from build123d import *

# Parameters (mm, degrees)
BOSS_EXTRUDE1_DEPTH        = 3
F_10_0MM_DOWEL_HOLE1_D     = 10
F_10_0MM_DOWEL_HOLE1_DEPTH = 3
F_3_0MM_DOWEL_HOLE1_D      = 3
F_3_0MM_DOWEL_HOLE1_DEPTH  = 3


with BuildPart() as part:
    # Sketch1 → Boss-Extrude1 (new body)
    with BuildSketch(Plane(origin=(0, 0, 0), x_dir=(1, 0, 0), z_dir=(0, 1, 0))):
        Polygon((-13.2, 0), (180, 0), (150.720058283, 100), (16.079941717, 100), align=None)
    extrude(amount=BOSS_EXTRUDE1_DEPTH)

    # Ø10.0mm Dowel Hole1
    with Locations(Plane(origin=(0, 3, 0), x_dir=(1, 0, 0), z_dir=(0, 1, 0))):
        with Locations((83.4, 50)):
            Hole(F_10_0MM_DOWEL_HOLE1_D / 2, depth=F_10_0MM_DOWEL_HOLE1_DEPTH)

    # Ø3.0mm Dowel Hole1
    with Locations(Plane(origin=(0, 3, 0), x_dir=(1, 0, 0), z_dir=(0, 1, 0))):
        with Locations((73.45, 58.95), (73.45, 41.05), (93.35, 41.05), (93.35, 58.95)):
            Hole(F_3_0MM_DOWEL_HOLE1_D / 2, depth=F_3_0MM_DOWEL_HOLE1_DEPTH)


solid = part.part
Model file for the job. Use its own axes, mm. Give positions to 0.01 mm unless a question says otherwise; leave off trailing zeros. Order: outer loops, then holes, each group sorted by start corner. A loop starts at its lowest first (then second) coordinate and runs counter-clockwise, first axis right, second up. Notation, with made-up numbers: (53.5, -34) - (109.5, -34) arc R21 cw to (109.5, -15) - close; hole circle Ø1 at (-12.75, 76.25). An arc over 180 degrees is marked (long way). Write item = value, one per line. Start each with the question number.
1. Probe line 1 along Z through (x, y) = (73.45, 1.7); line 2 along X through (y, z) = (1.25, -41.05); line 3 along Z through (x, y) = (83.4, 1.15). List the from-to ranges inside material, lowest first.
2. Two-plate mould, pull along Z, no slides. Class faces 1 (the flat face through (1.645, 1.479, -50.7)), 2 (the flat face through (82, 0, -40)), 3 (the cylindrical face through (80.712, 1.479, -54.216)): pulls with the +Z half, pulls with the -Z half, needs draft (parallel to the pull), parting line crosses it, or undercut.
3. Cut at A-A, the plane y = 0.5. List the corners of the cut face in (x, z).
4. Drop a flat-ended pin along its axis: P1, Ø1.8, axis at x = 73.45, z = -58.95, coming from the -Y side. Give the stop position or say it passes through.
5. Cut at C-C, the plane z = -75. List the corners of the cut face in (x, y).
6. Cut at B-B, the plane z = -50. List the corners of the cut face in (x, y).
Taken from the geometry:
q1.line_1 = -100 to -60.45, -57.45 to -42.55, -39.55 to 0
q1.line_2 = -1.18 to 71.95, 74.95 to 91.85, 94.85 to 167.98
q1.line_3 = -100 to -55, -45 to 0
q2.face_1 = pulls with the -Z half
q2.face_2 = needs draft
q2.face_3 = undercut
q3.outline = (-13.2, 0) - (16.08, -100) - (150.72, -100) - (180, 0) - close; hole circle Ø3 at (73.45, -58.95); hole circle Ø3 at (73.45, -41.05); hole circle Ø10 at (83.4, -50); hole circle Ø3 at (93.35, -58.95); hole circle Ø3 at (93.35, -41.05)
q4.P1 = through
q5.outline = (8.76, 0) - (158.04, 0) - (158.04, 3) - (8.76, 3) - close
q6.outline = (1.44, 0) - (78.4, 0) - (78.4, 3) - (1.44, 3) - close; (88.4, 0) - (165.36, 0) - (165.36, 3) - (88.4, 3) - close
